Input: part model. Units: mm. Frame: model coordinates. Face numbers are marked on the shaded views. A direction names the side the tool comes from. Coordinates: 2 decimals unless noted, no trailing zeros. Write each loop counter-clockwise with the first axis right and the second up, starting at its lowest first coordinate (ties: lowest second). Pieces come first, ordered by that corner, then holes.
1) Section query D-D (z = 10.25). Output: boundary loops of the cut face in (x, y), then the cut area to 3 significant figures.
2) Draft query along Y for the marked faces 4, 5 and 6. Return one class per face: pulls with the +Y half, pulls with the -Y half, needs draft (parallel to the pull), parting line crosses it, or undercut.
3) Section query B-B (z = 15.5). Output: boundary loops of the cut face in (x, y), then the cut area to 3 significant figures.
4) Pin query (flat end, axial travel): pin 1 Ø3 at (x, y) = (-8.5, -5) entering from +Z; pin 2 Ø1 at (x, y) = (2, 3.5) entering from -Z; pin 3 Ø3 at (x, z) = (4.5, 17) entering from +Y; pin 4 Ø0.9 at (y, z) = (-13.5, 16.5) entering from +X. Return the tip coordinate at first contact, or that it passes through.
5) Section query A-A (x = 0). Output: boundary loops of the cut face in (y, z), then the cut area to 4 significant figures.
6) Set-up query: the marked faces 1, 2 and 3. Return all of +Z, -Z, +X, -X, +Y, -Y with unobstructed straight access to the full face (end or side cutting, diameter ignored); none if empty.
7) Line query: L1, parallel to Z at x = 4.5, y = -5.5; L2, parallel to X at y = -11, z = 17.25; L3, parallel to Y at x = 8.75, z = 5. Output: solid intervals per line, ascending.
8) Section query C-C (y = 1). Output: boundary loops of the cut face in (x, z).
from build123d import *

# Parameters (mm, degrees)
BOSS_EXTRU_1_DEPTH = 14.5
CHANFREIN1_SIZE    = 2
ESQUISSE2_W        = 22
ESQUISSE2_H        = 7.5
BOSS_EXTRU_2_DEPTH = 6
BOSS_EXTRU_3_DEPTH = 3


with BuildPart() as part:
    # Esquisse1 → Boss.-Extru.1 (new body)
    with BuildSketch(Plane.XY):
        with BuildLine():
            Line((-11, 0), (-11, -23))
            Line((-11, -23), (11, -23))
            Line((11, -23), (11, 0))
            ThreePointArc((11, 0), (0, 11), (-11, 0))
        make_face()
    extrude(amount=BOSS_EXTRU_1_DEPTH)

    # Chanfrein1
    chanfrein1_edges = [part.edges().sort_by_distance(p)[0] for p in [
        (0, -23, 0),
    ]]
    chamfer(chanfrein1_edges, length=CHANFREIN1_SIZE)

    # Esquisse2 → Boss.-Extru.2 (add)
    with BuildSketch(Plane.XY.offset(14.5)):
        with Locations((0, -19.25)):
            Rectangle(ESQUISSE2_W, ESQUISSE2_H)
    extrude(amount=BOSS_EXTRU_2_DEPTH)

    # Esquisse3 → Boss.-Extru.3 (add)
    with BuildSketch(Plane.XY.offset(14.5)):
        with BuildLine():
            Line((-5, -9.797958971), (-5, -15.5))
            Line((-5, -15.5), (5, -15.5))
            Line((5, -15.5), (5, -9.797958971))
            ThreePointArc((5, -9.797958971), (0, 11), (-5, -9.797958971))
        make_face()
    extrude(amount=BOSS_EXTRU_3_DEPTH)


solid = part.part
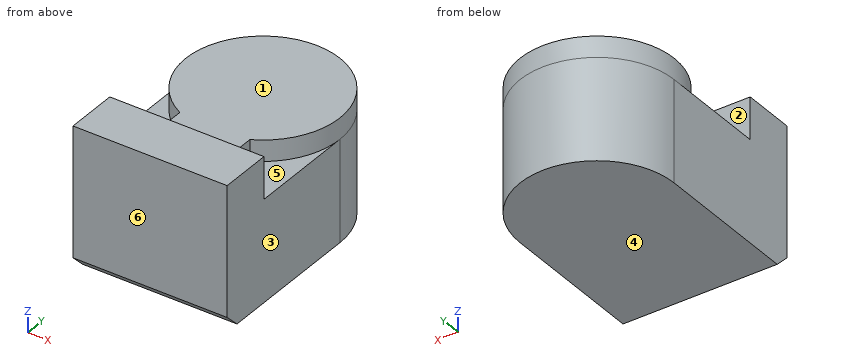
Answer:
1. outline: (-11, -23) - (11, -23) - (11, 0) arc R11 ccw to (-11, 0) - close
1. area: 696 mm2
2. face 4: needs draft
2. face 5: undercut
2. face 6: pulls with the -Y half
3. outline: (-11, -23) - (11, -23) - (11, -15.5) - (5, -15.5) - (5, -9.8) arc R11 ccw (long way) to (-5, -9.8) - (-5, -15.5) - (-11, -15.5) - close
3. area: 594 mm2
4. pin 1: stops at z = 17.5
4. pin 2: stops at z = 0
4. pin 3: stops at y = 10.58
4. pin 4: stops at x = 5
5. outline: (-23, 2) - (-21, 0) - (11, 0) - (11, 17.5) - (-15.5, 17.5) - (-15.5, 20.5) - (-23, 20.5) - close
5. area: 615.5 mm2
6. face 1: +Z, +X, -X, +Y
6. face 2: +Z
6. face 3: +Z, -Z, +X, +Y, -Y
7. L1: z = 0 to 17.5
7. L2: x = -5 to 5
7. L3: y = -23 to 6.67
8. outline: (-10.95, 0) - (10.95, 0) - (10.95, 17.5) - (-10.95, 17.5) - close
